Part model, mm, in its own coordinate system. A direction names the side the tool comes from. Round coordinates to 2 decimals unless told otherwise and drop trailing zeros. Loops run counter-clockwise (first coordinate to the right, second up) from the corner with the lowest first, then second, coordinate; pieces in that order, holes last. Notation, with made-up numbers: (36, -15.75) - (80, -15.75) arc R7 ccw to (80, -6.75) - close; hole circle Ø4 at (-11.75, -29). An arc over 180 degrees is marked (long way). Put each result on its own line as item: value.
from build123d import *

# Parameters (mm, degrees)
BOX036_W                = 2
BOX036_H                = 6
BOX036_DEPTH            = 10
CYLINDER030_R           = 1.6
CYLINDER030_DEPTH       = 50
CYLINDER029_R           = 5
CYLINDER029_DEPTH       = 22.5
CYLINDER031_R           = 1.6
CYLINDER031_DEPTH       = 50
CYLINDER019_R           = 1.6
CYLINDER019_DEPTH       = 40
CYLINDER019_PITCH_ANGLE = 90
CYLINDER018_R           = 1.6
CYLINDER018_DEPTH       = 40
CYLINDER018_PITCH_ANGLE = 90
CYLINDER017_R           = 1.6
CYLINDER017_DEPTH       = 40
CYLINDER016_R           = 1.6
CYLINDER016_DEPTH       = 70
CYLINDER016_ROLL_ANGLE  = 90
CYLINDER015_R           = 1.6
CYLINDER015_DEPTH       = 40
BOX012_W                = 116
BOX012_H                = 45
BOX012_DEPTH            = 5


with BuildPart() as cube024:
    # Box036 → Box036 (new body)
    with BuildSketch(Plane(origin=(64, 0, -8), x_dir=(1, 0, 0), z_dir=(0, 0, 1))):
        with Locations((1, 3)):
            Rectangle(BOX036_W, BOX036_H)
    extrude(amount=BOX036_DEPTH)


with BuildPart() as cylinder030:
    # Cylinder030 → Cylinder030 (new body)
    with BuildSketch(Plane(origin=(20.4, 8.8, -22), x_dir=(1, 0, 0), z_dir=(0, 0, 1))):
        Circle(CYLINDER030_R)
    extrude(amount=CYLINDER030_DEPTH)


with BuildPart() as fusion034:
    # Cylinder029 → Cylinder029 (new body)
    with BuildSketch(Plane.XY.offset(-12)):
        Circle(CYLINDER029_R)
    extrude(amount=CYLINDER029_DEPTH)

    # Fusion034: union Cylinder030
    add(cylinder030.part)


with BuildPart() as motor_holes_z:
    # Cylinder031 → Cylinder031 (new body)
    with BuildSketch(Plane(origin=(20.4, -8.8, -22), x_dir=(1, 0, 0), z_dir=(0, 0, 1))):
        Circle(CYLINDER031_R)
    extrude(amount=CYLINDER031_DEPTH)

    # Fusion035: union Fusion034
    add(fusion034.part)


with BuildPart() as cylinder100:
    # Cylinder019 → Cylinder019 (new body)
    with BuildSketch(Plane.XY):
        Circle(CYLINDER019_R)
    extrude(amount=CYLINDER019_DEPTH)


with BuildPart() as cylinder100_1:
    # Cylinder019 pitch: moved
    add(cylinder100.part.rotate(Axis((0, 0, 0), (0, 1, 0)), CYLINDER019_PITCH_ANGLE))


with BuildPart() as cylinder100_2:
    # Cylinder019 placement: moved
    add(cylinder100_1.part.moved(Location((-40, 12, 9.5))))


with BuildPart() as fusion011:
    # Cylinder018 → Cylinder018 (new body)
    with BuildSketch(Plane.XY):
        Circle(CYLINDER018_R)
    extrude(amount=CYLINDER018_DEPTH)


with BuildPart() as fusion011_1:
    # Cylinder018 pitch: moved
    add(fusion011.part.rotate(Axis((0, 0, 0), (0, 1, 0)), CYLINDER018_PITCH_ANGLE))


with BuildPart() as fusion011_2:
    # Cylinder018 placement: moved
    add(fusion011_1.part.moved(Location((-40, -7, 2.5))))

    # Fusion011: union Cylinder100
    add(cylinder100_2.part)


with BuildPart() as fusion012:
    # Cylinder017 → Cylinder017 (new body)
    with BuildSketch(Plane(origin=(-27.5, 7, -15), x_dir=(1, 0, 0), z_dir=(0, 0, 1))):
        Circle(CYLINDER017_R)
    extrude(amount=CYLINDER017_DEPTH)

    # Fusion012: union Fusion011
    add(fusion011_2.part)


with BuildPart() as fusion013:
    # Cylinder016 → Cylinder016 (new body)
    with BuildSketch(Plane.XY):
        Circle(CYLINDER016_R)
    extrude(amount=CYLINDER016_DEPTH)


with BuildPart() as fusion013_1:
    # Cylinder016 roll: moved
    add(fusion013.part.rotate(Axis((0, 0, 0), (1, 0, 0)), CYLINDER016_ROLL_ANGLE))


with BuildPart() as fusion013_2:
    # Cylinder016 placement: moved
    add(fusion013_1.part.moved(Location((-24, 39, 6))))

    # Fusion013: union Fusion012
    add(fusion012.part)


with BuildPart() as cylinder008:
    # Cylinder015 → Cylinder015 (new body)
    with BuildSketch(Plane(origin=(-20.5, -12, -15), x_dir=(1, 0, 0), z_dir=(0, 0, 1))):
        Circle(CYLINDER015_R)
    extrude(amount=CYLINDER015_DEPTH)


with BuildPart() as face_corner_holes008:
    # Fusion022 base: copy of Cylinder008
    add(cylinder008.part)

    # Fusion022: union Fusion013
    add(fusion013_2.part)


with BuildPart() as face_corner_holes008_1:
    # Fusion022 placement: moved
    add(face_corner_holes008.part.moved(Location((104, 0, 0))))


with BuildPart() as face_corner_holes005:
    # Fusion019 base: copy of Cylinder008
    add(cylinder008.part)

    # Fusion019: union Fusion013
    add(fusion013_2.part)


with BuildPart() as left_a:
    # Box012 → Box012 (new body)
    with BuildSketch(Plane(origin=(-30, -23, -5), x_dir=(1, 0, 0), z_dir=(0, 0, 1))):
        with Locations((58, 22.5)):
            Rectangle(BOX012_W, BOX012_H)
    extrude(amount=BOX012_DEPTH)

    # Cut014: cut face-corner-holes005
    add(face_corner_holes005.part, mode=Mode.SUBTRACT)

    # Cut018: cut face-corner-holes008
    add(face_corner_holes008_1.part, mode=Mode.SUBTRACT)

    # Cut029: cut motor-holes-z
    add(motor_holes_z.part, mode=Mode.SUBTRACT)

    # Cut061: cut Cube024
    add(cube024.part, mode=Mode.SUBTRACT)


solid = left_a.part
1. Two-plate mould, pull along X, no slides. Class faces 1 (the cylindrical face through (21.88, -9.41, -2.54)), 2 (the flat face through (27, 0, -5)), 3 (the flat face through (-30, -1, -3)): pulls with the +X half, pulls with the -X half, needs draft (parallel to the pull), parting line crosses it, or undercut.
A:
face 1: undercut
face 2: needs draft
face 3: pulls with the -X half
2. Probe line 1 along X through (y, z) = (-12, -3.4); line 2 along X through (y, z) = (7, -1.4); line 3 along Y through (x, z) = (-27.5, -3.35). List the from-to ranges inside material, lowest first. Write a range as [from, to].
A:
line 1: x = [-30, -22.1], [-18.9, 81.9], [85.1, 86]
line 2: x = [-30, -29.1], [-25.9, 74.9], [78.1, 86]
line 3: y = [-23, 5.4], [8.6, 22]
3. Tool access for faces 4 (the flat face through (86, -1, -3)), 5 (the flat face through (65, 6, -3)): list every direction of +Z, -Z, +X, -X, +Y, -Y with a clear straight run to the whole face (end or side of a thin tool).
A:
face 4: +Z, -Z, +X, +Y, -Y
face 5: +Z, -Z
4. Band-saw the part on C-C (x = 20.4). List the corners of the cut face in (y, z), plus the area to 3 significant figures.
A:
outline: (-23, -5) - (-10.4, -5) - (-10.4, 0) - (-23, 0) - close; (-7.2, -5) - (7.2, -5) - (7.2, 0) - (-7.2, 0) - close; (10.4, -5) - (22, -5) - (22, 0) - (10.4, 0) - close
area: 193 mm²
5. Band-saw the part on B-B (y = 4). List the corners of the cut face in (x, z).
A:
outline: (-30, -5) - (-3, -5) - (-3, 0) - (-30, 0) - close; (3, -5) - (64, -5) - (64, 0) - (3, 0) - close; (66, -5) - (86, -5) - (86, 0) - (66, 0) - close
6. Band-saw the part on D-D (z = -3.9). Give the number of separate pieces and of enclosed holes in the cut face, plus the area to 3 significant figures.
A:
separate pieces: 1
enclosed holes: 8
area: 5,080 mm²
7. Band-saw the part on A-A (x = 0). List the corners of the cut face in (y, z), plus the area to 3 significant figures.
A:
outline: (-23, -5) - (-5, -5) - (-5, 0) - (-23, 0) - close; (5, -5) - (22, -5) - (22, 0) - (5, 0) - close
area: 175 mm²
